```python
from build123d import *

# Parameters (mm, degrees)
SKETCH1_W           = 42.5
SKETCH1_H           = 40
BOSS_EXTRUDE1_DEPTH = 2
SKETCH2_R           = 1.5
CUT_EXTRUDE1_DEPTH  = 4
SKETCH3_R           = 11
CUT_EXTRUDE2_DEPTH  = 4
SKETCH4_W           = 42.5
SKETCH4_H           = 4
BOSS_EXTRUDE2_DEPTH = 15


with BuildPart() as part:
    # Sketch1 → Boss-Extrude1 (new, symmetric)
    with BuildSketch(Plane.XY):
        Rectangle(SKETCH1_W, SKETCH1_H)
    extrude(amount=BOSS_EXTRUDE1_DEPTH, both=True)

    # Sketch2 → Cut-Extrude1 (cut)
    with BuildSketch(Plane(origin=(0, 0, -2), x_dir=(-1, 0, 0), z_dir=(0, 0, -1))):
        with Locations((-16.75, 15.5)):
            Circle(SKETCH2_R)
        with Locations((13.25, 15.5)):
            Circle(SKETCH2_R)
        with Locations((13.25, -14.5)):
            Circle(SKETCH2_R)
        with Locations((-16.75, -14.5)):
            Circle(SKETCH2_R)
    extrude(amount=-CUT_EXTRUDE1_DEPTH, mode=Mode.SUBTRACT)

    # Sketch3 → Cut-Extrude2 (cut)
    with BuildSketch(Plane.XY.offset(2)):
        with Locations((1.25, 0)):
            Circle(SKETCH3_R)
    extrude(amount=-CUT_EXTRUDE2_DEPTH, mode=Mode.SUBTRACT)

    # Sketch4 → Boss-Extrude2 (add)
    with BuildSketch(Plane(origin=(0, 20, 0), x_dir=(1, 0, 0), z_dir=(0, 1, 0))):
        Rectangle(SKETCH4_W, SKETCH4_H)
    extrude(amount=BOSS_EXTRUDE2_DEPTH)


solid = part.part
```
Check sheet for the modelled part. Datum: model origin and axes. Units: mm. Give positions to 0.01 mm unless a question says otherwise; leave off trailing zeros. Write each loop counter-clockwise with the first axis right and the second up, starting at its lowest first coordinate (ties: lowest second). Pieces come first, ordered by that corner, then holes. Notation, with made-up numbers: (-31, 20.5) - (13, 20.5) arc R29 ccw to (13, 48.5) - close; hole circle Ø3 at (38.25, 20). An arc over 180 degrees is marked (long way). Answer as a JSON object with one key per item and string values. Group by question number.
1) Sectioned sample at B-B (x = 16.75). Record the cut outline in (y, z), then the cut area to 3 significant figures.
2) Sectioned sample at A-A (y = -14.5). Record the cut outline in (x, z).
3) Release check for a two-part mould opening along X. For faces 1 (the face through (21.25, 7, 0)), 2 (the face through (18.25, 15.57, -0.03)), 3 (the face through (-11.75, -14.43, -0.03)), 4 (the face through (-21.25, 7, 0)) record: pulls with the +X half, pulls with the -X half, needs draft (parallel to the pull), parting line crosses it, or undercut.
4) Thickness scan on probe 1 along Y at (x, z) = (16.75, 0); probe 2 along Y at (x, z) = (1.25, -0.45); probe 3 along X at (y, z) = (16, 1.2). Record the ranges inside material, lowest first. Write a range as from..to.
5) Sectioned sample at D-D (y = 0). Record the cut outline in (x, z).
6) Sectioned sample at C-C (z = -0.35). Record the cut outline in (x, y).
Geometry results:
{
 "1": {"outline": "(-20, -2) - (-16, -2) - (-16, 2) - (-20, 2) - close; (-13, -2) - (14, -2) - (14, 2) - (-13, 2) - close; (17, -2) - (35, -2) - (35, 2) - (17, 2) - close", "area": "196 mm^2"},
 "2": {"outline": "(-21.25, -2) - (-14.75, -2) - (-14.75, 2) - (-21.25, 2) - close; (-11.75, -2) - (15.25, -2) - (15.25, 2) - (-11.75, 2) - close; (18.25, -2) - (21.25, -2) - (21.25, 2) - (18.25, 2) - close"},
 "3": {"face 1": "pulls with the +X half", "face 2": "undercut", "face 3": "undercut", "face 4": "pulls with the -X half"},
 "4": {"probe 1": "y = -20..-16, -13..14, 17..35", "probe 2": "y = -20..-11, 11..35", "probe 3": "x = -21.25..-14.66, -11.84..15.34, 18.16..21.25"},
 "5": {"outline": "(-21.25, -2) - (-9.75, -2) - (-9.75, 2) - (-21.25, 2) - close; (12.25, -2) - (21.25, -2) - (21.25, 2) - (12.25, 2) - close"},
 "6": {"outline": "(-21.25, -20) - (21.25, -20) - (21.25, 35) - (-21.25, 35) - close; hole circle Ø3 at (-13.25, -14.5); hole circle Ø3 at (-13.25, 15.5); hole circle Ø22 at (1.25, 0); hole circle Ø3 at (16.75, -14.5); hole circle Ø3 at (16.75, 15.5)"}
}
